Geometry check sheet. Reference: drawing and pictorial views, mm from the part's lowest x, y, z. Round coordinates to 2 decimals unless told otherwise and drop trailing zeros. Write each loop counter-clockwise with the first axis right and the second up, starting at its lowest first coordinate (ties: lowest second). Pieces come first, ordered by that corner, then holes.
Item 1: Section check C-C, the plane y = 4.55. Record the cut outline in (x, z).
Item 2: Section check B-B, the plane x = 29.21. Record the cut outline in (y, z), plus the area to 3 significant figures.
Item 3: Depth check by flat-ended pin: pin 1 (2.5 mm diameter, centred on x = 30, y = 3.5, fed in from +Z); pin 2 (1 mm diameter, centred on y = 3.5, z = 42.5, fed in from +X); pin 3 (3 mm diameter, centred on y = 5, z = 45, fed in from +X). Enter the tip coordinate at first touch or a pass-through.
Item 4: Material ranges on line 1 along Z through (x, y) = (28.5, 2.7); line 2 along Z through (x, y) = (27, 1.15); line 3 along X through (y, z) = (0.9, 22), recorded low to high.
Item 5: Section check D-D, the plane z = 5. Record the cut outline in (x, y), plus the area to 3 significant figures.
Item 6: Section check A-A, the plane z = 29.21. Record the cut outline in (x, y).
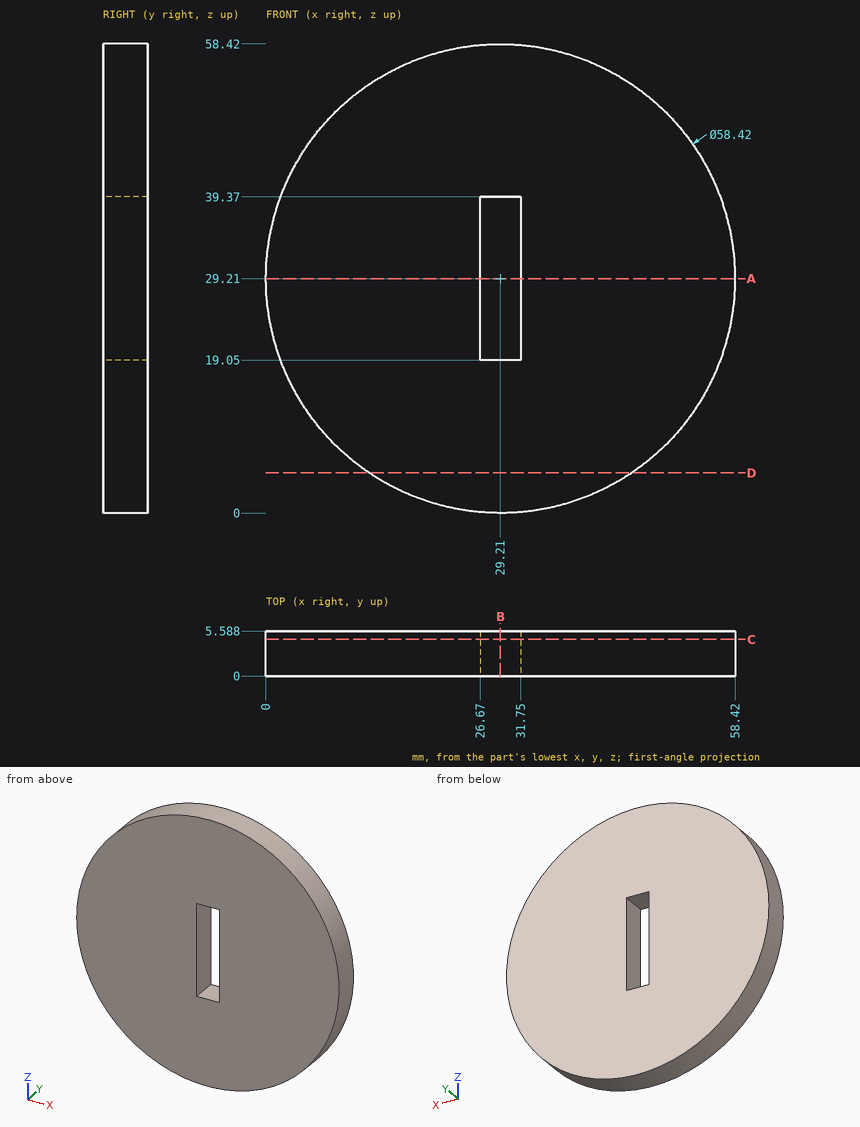
Values found:
1. outline: circle Ø58.42 at (29.21, 29.21); hole (26.67, 19.05) - (31.75, 19.05) - (31.75, 39.37) - (26.67, 39.37) - close
2. outline: (0, 0) - (5.59, 0) - (5.59, 19.05) - (0, 19.05) - close; (0, 39.37) - (5.59, 39.37) - (5.59, 58.42) - (0, 58.42) - close
2. area: 213 mm2
3. pin 1: stops at z = 58.42
3. pin 2: stops at x = 55.47
3. pin 3: stops at x = 54.69
4. line 1: z = 0.01 to 19.05, 39.37 to 58.41
4. line 2: z = 0.08 to 19.05, 39.37 to 58.34
4. line 3: x = 0.9 to 26.67, 31.75 to 57.52
5. outline: (12.87, 0) - (45.55, 0) - (45.55, 5.59) - (12.87, 5.59) - close
5. area: 183 mm2
6. outline: (0, 0) - (26.67, 0) - (26.67, 5.59) - (0, 5.59) - close; (31.75, 0) - (58.42, 0) - (58.42, 5.59) - (31.75, 5.59) - close
